from build123d import *

# Parameters (mm, degrees)
F0_W     = 15
F0_H     = 15
F1_DEPTH = 62.5
F3_R     = 6
F4_R     = 6
F2_R     = 4
F5_DEPTH = 30
F6_R     = 4
F7_DEPTH = 30
F9_D     = 5
F10_R    = 2
F11_R    = 2


with BuildPart() as f1:
    # F0 (on Top) → F1 (new body)
    with BuildSketch(Plane.XY):
        Rectangle(F0_W, F0_H)
    extrude(amount=F1_DEPTH)

    # F3
    f3_edges = [f1.edges().sort_by_distance(p)[0] for p in [
        (0, -7.5, 62.5),
    ]]
    fillet(f3_edges, radius=F3_R)

    # F4
    f4_edges = [f1.edges().sort_by_distance(p)[0] for p in [
        (0, 7.5, 62.5),
    ]]
    fillet(f4_edges, radius=F4_R)

    # F2 (on face) → F5 (join)
    with BuildSketch(Plane(origin=(-7.5, 0, 0), x_dir=(0, -1, 0), z_dir=(-1, 0, 0))):
        with Locations((0, 55.5)):
            Circle(F2_R)
    extrude(amount=F5_DEPTH)

    # F6 (on face) → F7 (join)
    with BuildSketch(Plane.YZ.offset(7.5)):
        with Locations((0, 55.5)):
            Circle(F6_R)
    extrude(amount=F7_DEPTH)

    # F9 (through all)
    with Locations(Plane(origin=(-7.5, 0, 0), x_dir=(0, -1, 0), z_dir=(-1, 0, 0))):
        with Locations((0, 6.25)):
            Hole(F9_D / 2)

    # F10
    f10_edges = [f1.edges().sort_by_distance(p)[0] for p in [
        (37.5, -4, 55.5),
    ]]
    fillet(f10_edges, radius=F10_R)

    # F11
    f11_edges = [f1.edges().sort_by_distance(p)[0] for p in [
        (-37.5, 4, 55.5),
    ]]
    fillet(f11_edges, radius=F11_R)


solid = f1.part
Could you check a few things on this model? Use its own coordinates, in mm. A direction names the side the tool comes from. Give positions to 0.01 mm unless a question says otherwise; leave off trailing zeros. Order: outer loops, then holes, each group sorted by start corner. A loop starts at its lowest first (then second) coordinate and runs counter-clockwise, first axis right, second up. Notation, with made-up numbers: (49.25, -38) - (108.25, -38) arc R20 cw to (108.25, -20) - close; hole circle Ø8 at (29.5, -25.75). An arc over 180 degrees is marked (long way). One line per question, with ' | ' between items. Start each with the question number.
Item 1: I want a section at C-C on x = 25. Write out the boundary of the cut face in (y, z).
Item 2: Thinking about a two-plate mould opening in Z: for faces 1 (the flat face through (0, 7.5, 28)), 2 (the flat face through (0, 0, 62.5)), 3 (the cylindrical face through (0.11, -0.33, 8.73)), which applies, pulls with the +Z half, pulls with the -Z half, needs draft (parallel to the pull), parting line crosses it, or undercut?
Item 3: I want a section at B-B on x = 4. Write out the boundary of the cut face in (y, z), then the cut area to 3 significant figures.
Item 4: I'm going to push flat-ended pins straight in: pin 1 Ø2 at (y, z) = (-4.5, 21.5) entering from -X; pin 2 Ø3 at (y, z) = (4, 18) entering from +X; pin 3 Ø4 at (x, y) = (19, -1.5) entering from -Z. Where does each tip first touch, or does it pass through?
Item 5: For faces 4 (the cylindrical face through (-21.304, 0.867, 51.595)), 5 (the cylindrical face through (0.105, 5.696, 60.789)), 6 (the cylindrical face through (21.304, -0.867, 51.595)), which set-ups out of +Z, -Z, +X, -X, +Y, -Y let a thin tool reach every point of the face, with its end or its side?
Item 6: I need wall thicknesses on probe 1 along Z at (x, y) = (-3, 0.25); probe 2 along X at (y, z) = (-6.25, 13); probe 3 along Y at (x, z) = (0, 7). Which ranges of each line are inside material? Lowest first, please. Write a range as [from, to].
Item 7: I want a section at A-A on z = 6.25. Write out the boundary of the cut face in (x, y), then the cut area to 3 significant figures.
Item 8: I want a section at D-D on y = -6.5. Write out the boundary of the cut face in (x, z), then the cut area to 3 significant figures.
Verdict:
1) outline: circle Ø8 at (0, 55.5)
2) face 1: needs draft | face 2: pulls with the +Z half | face 3: undercut
3) outline: (-7.5, 0) - (7.5, 0) - (7.5, 56.5) arc R6 ccw to (1.5, 62.5) - (-1.5, 62.5) arc R6 ccw to (-7.5, 56.5) - close; hole circle Ø5 at (0, 6.25) | area: 902 mm^2
4) pin 1: x = -7.5 | pin 2: x = 7.5 | pin 3: z = 51.5
5) face 4: -X | face 5: +Z, +X, -X, +Y | face 6: +X
6) probe 1: [0, 3.76], [8.74, 62.5] | probe 2: [-7.5, 7.5] | probe 3: [-7.5, -2.38], [2.38, 7.5]
7) outline: (-7.5, -7.5) - (7.5, -7.5) - (7.5, -2.5) - (-7.5, -2.5) - close; (-7.5, 2.5) - (7.5, 2.5) - (7.5, 7.5) - (-7.5, 7.5) - close | area: 150 mm^2
8) outline: (-7.5, 0) - (7.5, 0) - (7.5, 59.82) - (-7.5, 59.82) - close | area: 897 mm^2
